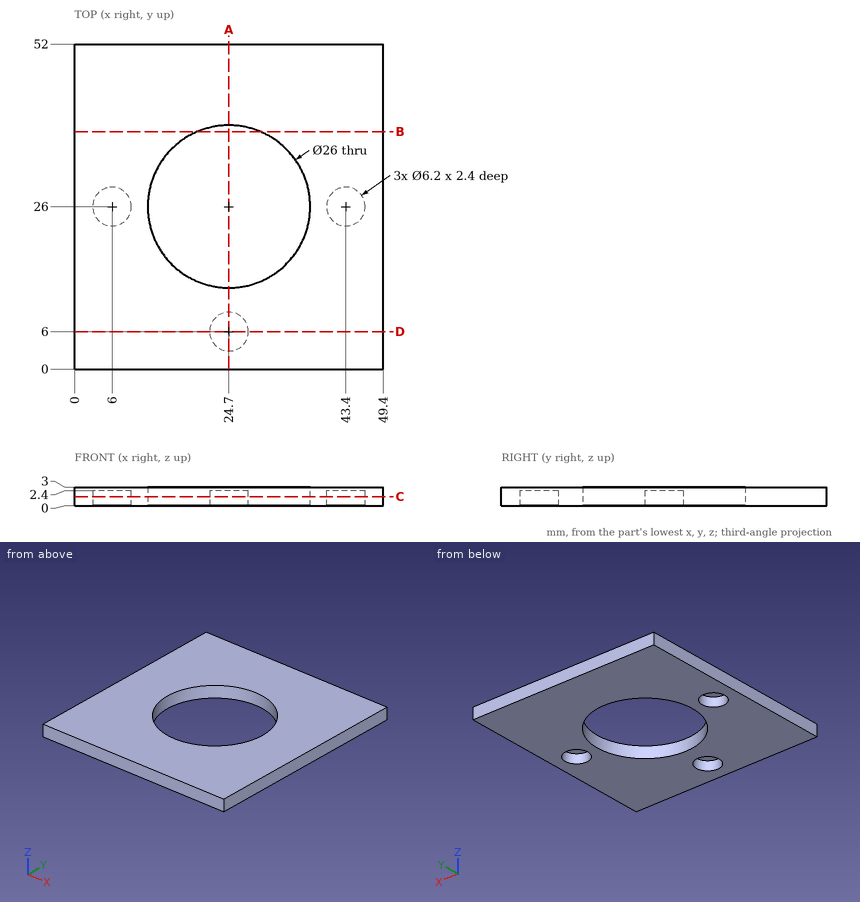
Drawing for the job (mm, zero at the part's lowest x, y, z). Coordinates: 2 decimals unless noted, no trailing zeros. Order: outer loops, then holes, each group sorted by start corner. A loop starts at its lowest first (then second) coordinate and runs counter-clockwise, first axis right, second up. Notation, with made-up numbers: (27, 25.25) - (80, 25.25) arc R28 cw to (80, 45.25) - close; hole circle Ø5 at (70.5, 8.5). An arc over 180 degrees is marked (long way). Use a Markdown table: item, result. Add a question column.
(1) Saw through at A-A (x = 24.7). Give the cut face in (y, z), then the cut area to 3 significant figures.
(2) Drill centre lines: line 1 along X through (y, z) = (27.5, 1.05); line 2 along Y through (x, z) = (24.7, 2.45); line 3 along Y through (x, z) = (6, 1.5). Where is each one in solid material? Low to high. Write a range as [from, to].
(3) Saw through at D-D (y = 6). Give the cut face in (x, z).
(4) Saw through at B-B (y = 38). Give the cut face in (x, z), then the cut area to 3 significant figures.
(5) Saw through at C-C (z = 1.5). Give the cut face in (x, y), then the cut area to 3 significant figures.
(6) Flat gauge pin, fed straight in: pin 1 (3 mm diameter, centred on x = 42.5, y = 25.5, fed in from -Z). Where does the tip first touch, or does it go through?
Solved:
| question | item | result |
|---|---|---|
| 1 | outline | (0, 0) - (2.9, 0) - (2.9, 2.4) - (9.1, 2.4) - (9.1, 0) - (13, 0) - (13, 3) - (0, 3) - close; (39, 0) - (52, 0) - (52, 3) - (39, 3) - close |
| 1 | area | 63.1 mm² |
| 2 | line 1 | x = [0, 3.29], [8.71, 11.79], [37.61, 40.69], [46.11, 49.4] |
| 2 | line 2 | y = [0, 13], [39, 52] |
| 2 | line 3 | y = [0, 22.9], [29.1, 52] |
| 3 | outline | (0, 0) - (21.6, 0) - (21.6, 2.4) - (27.8, 2.4) - (27.8, 0) - (49.4, 0) - (49.4, 3) - (0, 3) - close |
| 4 | outline | (0, 0) - (19.7, 0) - (19.7, 3) - (0, 3) - close; (29.7, 0) - (49.4, 0) - (49.4, 3) - (29.7, 3) - close |
| 4 | area | 118 mm² |
| 5 | outline | (0, 0) - (49.4, 0) - (49.4, 52) - (0, 52) - close; hole circle Ø6.2 at (6, 26); hole circle Ø26 at (24.7, 26); hole circle Ø6.2 at (24.7, 6); hole circle Ø6.2 at (43.4, 26) |
| 5 | area | 1,950 mm² |
| 6 | pin 1 | stops at z = 2.4 |
